Geometry check sheet. Reference: drawing and pictorial views, mm from the part's lowest x, y, z. Give positions to 0.01 mm unless a question says otherwise; leave off trailing zeros. Order: outer loops, then holes, each group sorted by start corner. A loop starts at its lowest first (then second) coordinate and runs counter-clockwise, first axis right, second up.
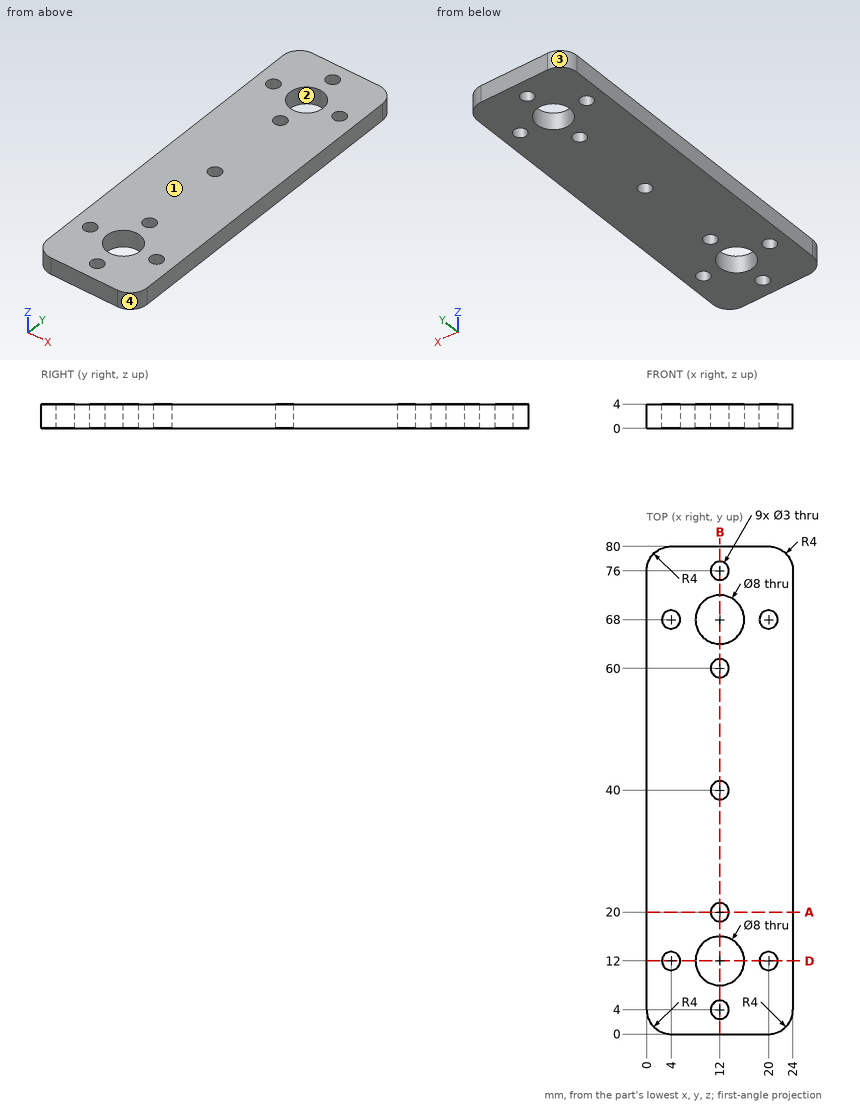
(1) Cross-section at A-A on y = 20. Enter the section's corners in (x, z).
Response values:
outline: (0, 0) - (10.5, 0) - (10.5, 4) - (0, 4) - close; (13.5, 0) - (24, 0) - (24, 4) - (13.5, 4) - close
(2) Cross-section at B-B on x = 12. Count the separate pieces of the cut face and the enclosed holes in it, then the cut area to 3 significant figures.
Response values:
separate pieces: 8
enclosed holes: 0
area: 196 mm2
(3) Release check for a two-part mould opening along Y. For the marked faces 1, 2, 3 and 4 record: released by +Y, released by -Y, zero draft, split by the parting line, or undercut.
Response values:
face 1: zero draft
face 2: undercut
face 3: released by +Y
face 4: released by -Y
(4) Cross-section at D-D on y = 12. Enter the section's corners in (x, z), then the cut area to 3 significant figures.
Response values:
outline: (0, 0) - (2.5, 0) - (2.5, 4) - (0, 4) - close; (5.5, 0) - (8, 0) - (8, 4) - (5.5, 4) - close; (16, 0) - (18.5, 0) - (18.5, 4) - (16, 4) - close; (21.5, 0) - (24, 0) - (24, 4) - (21.5, 4) - close
area: 40.0 mm2
(5) Gauge pin test, flat end, axial feed: pin 1 Ø2.5 at (x, y) = (12, 76) entering from +Z. Record the tip position at first contact, or that the pin passes through.
Response values:
pin 1: passes through
(6) Material ranges on L1, parallel to Y at x = 4, z = 0.9; L2, parallel to X at y = 13, z = 1.6; L3, parallel to X at y = 76, z = 2.1, recorded low to high.
Response values:
L1: y = 0 to 10.5, 13.5 to 66.5, 69.5 to 80
L2: x = 0 to 2.88, 5.12 to 8.13, 15.87 to 18.88, 21.12 to 24
L3: x = 0 to 10.5, 13.5 to 24
